Can you work these out from the model? Positions are in its coordinate system, mm. A direction names the side the tool comes from. Round coordinates to 2 decimals unless told otherwise and drop trailing zeros. Loops run counter-clockwise (first coordinate to the right, second up) from the corner with the lowest first, then second, coordinate; pieces in that order, holes last.
```python
from build123d import *

# Parameters (mm, degrees)
F1_DEPTH = 10
F3_R     = 1.7
F4_DEPTH = 25
F2_R     = 1.7
F5_DEPTH = 25


with BuildPart() as f1:
    # F0 (on Top) → F1 (new body)
    with BuildSketch(Plane.XY):
        Polygon((0, 3), (0, 0), (30, 0), (30, 30), (27, 30), (27, 3), align=None)
    extrude(amount=F1_DEPTH)

    # F3 (on face) → F4 (cut)
    with BuildSketch(Plane(origin=(27, 0, 0), x_dir=(0, -1, 0), z_dir=(-1, 0, 0))):
        with Locations((-25, 5)):
            Circle(F3_R)
        with Locations((-15, 5)):
            Circle(F3_R)
    extrude(amount=-F4_DEPTH, mode=Mode.SUBTRACT)

    # F2 (on face) → F5 (cut)
    with BuildSketch(Plane(origin=(0, 3, 0), x_dir=(-1, 0, 0), z_dir=(0, 1, 0))):
        with Locations((-15, 5)):
            Circle(F2_R)
        with Locations((-5, 5)):
            Circle(F2_R)
    extrude(amount=-F5_DEPTH, mode=Mode.SUBTRACT)


solid = f1.part
```
(1) Suppose I cut it at B-B (x = 5). Write out the boundary of the cut face in (y, z), then the cut area to 3 significant figures.
(2) For pin 1 (4 mm diameter, centred on y = 25, z = 5, fed in from -X); pin 2 (1 mm diameter, centred on x = 18, z = 3.5, fed in from +Y); pin 3 (10 mm diameter, centred on x = 24.5, y = 8, fed in from +Z), each with a flat end and sliding along its axis, tell me the tip position at first contact or that it passes through.
(3) Suppose I cut it at C-C (z = 5). Write out the boundary of the cut face in (x, y).
(4) Which directions (+Z, -Z, +X, -X, +Y, -Y) give clear straight access to the entire face, cutting with the end or side of a thin tool? Please do faces 4 (the flat face through (27, 17, 4)), 5 (the flat face through (21.6, 2.8, 0)).
(5) Suppose I cut it at D-D (z = 0.5). Write out the boundary of the cut face in (x, y).
(6) Suppose I cut it at A-A (y = 25). Write out the boundary of the cut face in (x, z).
(7) We'd pull the mould along Y, two halves only. Please class faces 1 (the cylindrical face through (28.48, 23.43, 4.35)), 2 (the flat face through (14, 3, 3)), 3 (the flat face through (21.6, 2.8, 10)): released by +Y, released by -Y, zero draft, split by the parting line, or undercut.
(8) If I drill on line 1 (Z direction, x = 29.25, y = 15); line 2 (X direction, y = 7.5, z = 0.5); line 3 (Y direction, x = 4, z = 3), over which ranges is the centre line in solid material (lowest first)?
Check result:
1. outline: (0, 0) - (3, 0) - (3, 3.3) - (0, 3.3) - close; (0, 6.7) - (3, 6.7) - (3, 10) - (0, 10) - close
1. area: 19.8 mm2
2. pin 1: stops at x = 27
2. pin 2: stops at y = 3
2. pin 3: stops at z = 10
3. outline: (0, 0) - (3.3, 0) - (3.3, 3) - (0, 3) - close; (6.7, 0) - (13.3, 0) - (13.3, 3) - (6.7, 3) - close; (16.7, 0) - (30, 0) - (30, 13.3) - (27, 13.3) - (27, 3) - (16.7, 3) - close; (27, 16.7) - (30, 16.7) - (30, 23.3) - (27, 23.3) - close; (27, 26.7) - (30, 26.7) - (30, 30) - (27, 30) - close
4. face 4: +Z, -Z, -X, +Y
4. face 5: -Z, +X, -X, +Y, -Y
5. outline: (0, 0) - (30, 0) - (30, 30) - (27, 30) - (27, 3) - (0, 3) - close
6. outline: (27, 0) - (30, 0) - (30, 3.3) - (27, 3.3) - close; (27, 6.7) - (30, 6.7) - (30, 10) - (27, 10) - close
7. face 1: undercut
7. face 2: released by +Y
7. face 3: zero draft
8. line 1: z = 0 to 3.3, 6.7 to 10
8. line 2: x = 27 to 30
8. line 3: y = 0 to 3
